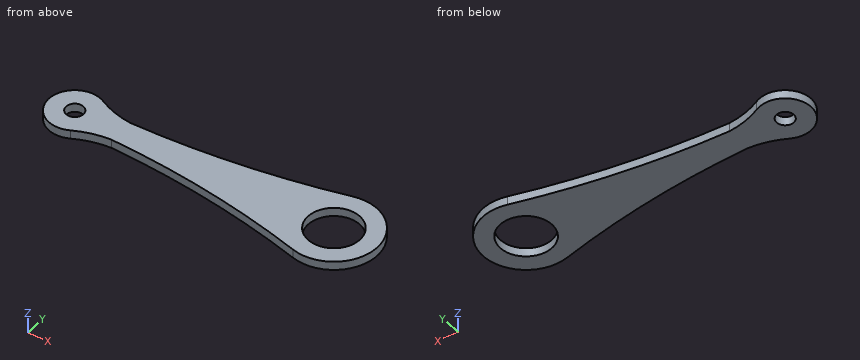
Autodesk Inventor part; units mm, degrees
ref_plane "YZ Plane" through (0, 0, 0) normal (1, 0, 0) x (0, 1, 0)
ref_plane "XZ Plane" through (0, 0, 0) normal (0, 1, 0) x (-1, 0, 0)
ref_plane "XY Plane" through (0, 0, 0) normal (0, 0, 1) x (1, 0, 0)
sketch "Эскиз1" plane through (0, 0, 0) normal (0, 0, 1) x (1, 0, 0)
  arc A0 (6.9948, 13.2692) -> (6.9948, -13.2692) centre (0, 0) ccw
  line L0 (30.3109, 7.5) -> (15.5799, 7.5)
  line L1 (30.3109, -7.5) -> (15.5799, -7.5)
  arc A1 (143.599, -24.1667) -> (143.599, 24.1667) centre (150, 0) ccw
  arc A2 (6.9948, 13.2692) -> (30.3109, 7.5) centre (30.3109, 57.5) ccw
  arc A3 (30.3109, -7.5) -> (6.9948, -13.2692) centre (30.3109, -57.5) ccw
  arc A4 (15.5799, 7.5) -> (143.599, 24.1667) centre (15.5799, 507.5) ccw
  arc A5 (143.599, -24.1667) -> (15.5799, -7.5) centre (15.5799, -507.5) ccw
  point P0 (12.9904, 7.5)
  point P1 (126.1515, 7.5)
  point P2 (12.9904, -7.5)
  point P3 (126.1515, -7.5)
  point P4 (-12.9904, 7.5)
  point P5 (-12.9904, -7.5)
  point P6 (126.1515, -7.5)
  point P7 (126.1515, 7.5)
  point P8 (12.9904, 7.5)
  point P9 (12.9904, -7.5)
  point P10 (26.7733, 7.6253)
  point P11 (26.7733, -7.6253)
  dimension "d0" = 30
  dimension "d1" = 50
  dimension "d5" = 150
  dimension "d17" = 15
  dimension "d19" = 50
  dimension "d20" = 500
extrude "Выдавливание1" add sketch "Эскиз1" along normal blind 5 contours A5 L1 A3 | A2 L0 A4 | A2 A4 A1 A5 A3 A0
sketch "Эскиз2" plane through (0, 0, 5) normal (0, 0, 1) x (1, 0, 0)
  arc A0 (143.599, -24.1667) -> (143.599, 24.1667) centre (150, 0) ccw
  point P0 (0, 0)
  point P1 (0, 0)
  point P2 (88.8197, -10)
  point P3 (88.8197, 10)
  point P4 (142.2738, -12.8571)
  point P5 (142.2738, 12.8571)
hole "Отверстие1" at (0, 0, 5) direction (0, 0, -1) diameter 10 end through all
sketch "Эскиз3" plane through (0, 0, 5) normal (0, 0, 1) x (1, 0, 0)
  arc A0 (143.599, -24.1667) -> (143.599, 24.1667) centre (150, 0) ccw
  point P0 (0, 0)
hole "Отверстие2" at (150, 0, 5) direction (0, 0, -1) diameter 30 end through all
properties part number "Рычаг_1"
Can you work these out from the model? Positions are in its coordinate system, mm. Give positions to 0.01 mm unless a question says otherwise; leave off trailing zeros. Order: outer loops, then holes, each group sorted by start corner. A loop starts at its lowest first (then second) coordinate and runs counter-clockwise, first axis right, second up. Notation, with made-up numbers: M 64,42.25 L 110,42.25 A29 cw 110,81.25 Z; hole C 72,-30.5 d3. An arc over 180 degrees is marked long. Write item = value, one per line. Start each with the question number.
Q1. I need wall thicknesses on probe 1 along X at (y, z) = (-0.5, 2.1); probe 2 along Y at (x, z) = (150, 1.6); probe 3 along Y at (x, z) = (0, 3.4). Which ranges of each line are inside material? Lowest first, please. Write a range as [from, to].
Q2. Suppose I cut it at C-C (y = 0). Write out the boundary of the cut face in (x, z).
Q3. Suppose I cut it at D-D (x = 75). Write out the boundary of the cut face in (y, z).
Q4. Suppose I cut it at A-A (x = 0). Write out the boundary of the cut face in (y, z).
Q5. Will these pins go through, and if not, where does the flat tip stop? pin 1 Ø2 at (y, z) = (-7, 3.5) entering from -X; pin 2 Ø1 at (x, z) = (119, 4.5) entering from -Y; pin 3 Ø2 at (x, z) = (7.5, 1) entering from +Y; pin 4 Ø1.5 at (x, y) = (10, -1) entering from -Z.
Q6. Suppose I cut it at B-B (z = 4). Write out the boundary of the cut face in (x, y).
Check result:
q1.probe_1 = [-14.99, -4.97], [4.97, 135.01], [164.99, 175]
q1.probe_2 = [-25, -15], [15, 25]
q1.probe_3 = [-15, -5], [5, 15]
q2.outline = M -15,0 L -5,0 L -5,5 L -15,5 Z; M 5,0 L 135,0 L 135,5 L 5,5 Z; M 165,0 L 175,0 L 175,5 L 165,5 Z
q3.outline = M -11.04,0 L 11.04,0 L 11.04,5 L -11.04,5 Z
q4.outline = M -15,0 L -5,0 L -5,5 L -15,5 Z; M 5,0 L 15,0 L 15,5 L 5,5 Z
q5.pin_1 = -13.75
q5.pin_2 = -18.42
q5.pin_3 = 13.52
q5.pin_4 = 0
q6.outline = M 6.99,-13.27 A50 cw 26.77,-7.63 A500 cw 143.6,-24.17 A25 ccw long 143.6,24.17 A500 cw 26.77,7.63 A50 cw 6.99,13.27 A15 ccw long Z; hole C 0,0 d10; hole C 150,0 d30
